Autodesk Inventor part; units mm, degrees
ref_plane "YZ Plane" through (0, 0, 0) normal (1, 0, 0) x (0, 1, 0)
ref_plane "XZ Plane" through (0, 0, 0) normal (0, 1, 0) x (-1, 0, 0)
ref_plane "XY Plane" through (0, 0, 0) normal (0, 0, 1) x (1, 0, 0)
sketch "Sketch1" plane through (0, 0, 0) normal (0, 0, 1) x (1, 0, 0)
  line L0 (-16, -12.5) -> (16, -12.5)
  line L1 (16, -12.5) -> (16, 12.5)
  line L2 (16, 12.5) -> (13, 12.5)
  line L3 (13, 12.5) -> (13, -9.5)
  line L4 (13, -9.5) -> (-13, -9.5)
  line L5 (-13, -9.5) -> (-13, 12.5)
  line L6 (-13, 12.5) -> (-16, 12.5)
  line L7 (-16, 12.5) -> (-16, -12.5)
  point P0 (0, 0)
  dimension "d0" = 32
  dimension "d1" = 25
  dimension "d2" = 3
  dimension "d3" = 90
  dimension "d4" = 22
  dimension "d5" = 26
  dimension "d6" = 22
  dimension "d7" = 3
  dimension "d8" = 25
  dimension "d10" = 12.5
  dimension "d11" = 16
extrude "Extrusion1" add sketch "Sketch1" against normal blind 609.6
chamfer "Chamfer1" distance 25 angle 30 1 edges at (14.5, 12.5, 0) measured on face at (4.3333, -11.5, 0)
chamfer "Chamfer2" distance 25 angle 30 1 edges at (14.5, 12.5, -609.6) measured on face at (4.3333, -11.5, -609.6)
sketch "Sketch2" plane through (16, -12.5, 0) normal (1, 0, 0) x (0, 0, -1)
  line L0 (595.1662, 25) -> (609.6, 0)
  line L1 (14.4338, 25) -> (595.1662, 25)
  line L2 (602.3831, 12.5) -> (599.0481, 12.5)
  line L3 (508, 12.5) -> (101.6, 12.5) construction
  line L4 (101.6, 12.5) -> (203.2, 12.5) construction
  line L5 (203.2, 12.5) -> (304.8, 12.5) construction
  line L6 (304.8, 12.5) -> (406.4, 12.5) construction
  line L7 (406.4, 12.5) -> (508, 12.5) construction
  circle A0 centre (101.6, 12.5) radius 3.175
  circle A1 centre (203.2, 12.5) radius 3.175
  circle A2 centre (304.8, 12.5) radius 3.175
  circle A3 centre (406.4, 12.5) radius 3.175
  circle A4 centre (508, 12.5) radius 3.175
  line L8 (0, 12.5) -> (609.6, 12.5) construction
  point P0 (0, 0)
  dimension "d21" = 3.335
  dimension "d23" = 406.4
  dimension "d24" = 101.6
  dimension "d25" = 101.6
  dimension "d26" = 101.6
  dimension "d28" = 6.35
  dimension "d29" = 6.35
  dimension "d30" = 6.35
  dimension "d31" = 6.35
  dimension "d32" = 6.35
  dimension "d35" = 101.6
  dimension "d36" = 609.6
  dimension "d37" = 101.6
  dimension "d38" = 101.6
hole "Mounting Holes" at (16, 0, -101.6) at (16, 0, -203.2) at (16, 0, -304.8) at (16, 0, -406.4) at (16, 0, -508) direction (-1, 0, 0) diameter 6.35 depth 8 tip angle 118
equation "\"d5\" = d0 - 2 * d2"
equation "\"d24\" = d35"
equation "\"d25\" = d24"
equation "\"d26\" = d24"
equation "\"d29\" = d28"
equation "\"d30\" = d28"
equation "\"d31\" = d28"
equation "\"d32\" = d28"
equation "\"d35\" = 0.166667 * d36"
equation "\"d37\" = d35"
properties part number "24in C-Channel"
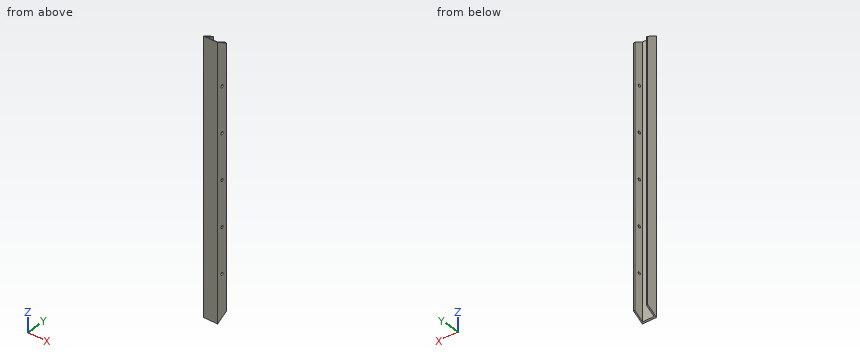
Geometry check sheet. Reference: the model listing, model coordinates, mm. Round coordinates to 2 decimals unless told otherwise and drop trailing zeros. Loops run counter-clockwise (first coordinate to the right, second up) from the corner with the lowest first, then second, coordinate; pieces in that order, holes last. Notation, with made-up numbers: (-35, -21) - (-16, -21) arc R12 ccw to (-16, -3) - close; hole circle Ø9 at (55, 72.5). An arc over 180 degrees is marked (long way). Use a Markdown table: item, result.
Q1. Material ranges on line 1 (X direction, y = -2.5, z = -514); line 2 (Y direction, x = 14.8, z = -304.8) (3 decimals); line 3 (Z direction, x = 13.8, y = 0) (3 decimals), recorded low to high.
Solutions:
| item | result |
|---|---|
| line 1 | x = -16 to -13, 13 to 16 |
| line 2 | y = -12.5 to -3.175, 3.175 to 12.5 |
| line 3 | z = -602.384 to -511.175, -504.825 to -409.575, -403.225 to -307.975, -301.625 to -206.375, -200.025 to -104.775, -98.425 to -7.216 |
Q2. Cross-section at B-B on z = -221. Record the cut outline in (x, y).
Solutions:
| item | result |
|---|---|
| outline | (-16, -12.5) - (16, -12.5) - (16, 12.5) - (13, 12.5) - (13, -9.5) - (-13, -9.5) - (-13, 12.5) - (-16, 12.5) - close |
Q3. Cross-section at A-A on y = 7.75. Record the cut outline in (x, z), plus the area to 3 significant figures.
Solutions:
| item | result |
|---|---|
| outline | (-16, -597.91) - (-13, -597.91) - (-13, -11.69) - (-16, -11.69) - close; (13, -597.91) - (16, -597.91) - (16, -11.69) - (13, -11.69) - close |
| area | 3,520 mm2 |
Q4. Go/stop test with flat-tipped pins: P1, Ø5.5, axis at y = 0, z = -203.2, coming from the +X side; P2, Ø13, axis at x = -2.5, z = -402, coming from the +Y side; P3, Ø6, axis at x = 10.5, y = 0, coming from the +Z side. Record where each tip stops, or that it passes through.
Solutions:
| item | result |
|---|---|
| P1 | stops at x = -13 |
| P2 | stops at y = -9.5 |
| P3 | stops at z = -6.26 |
